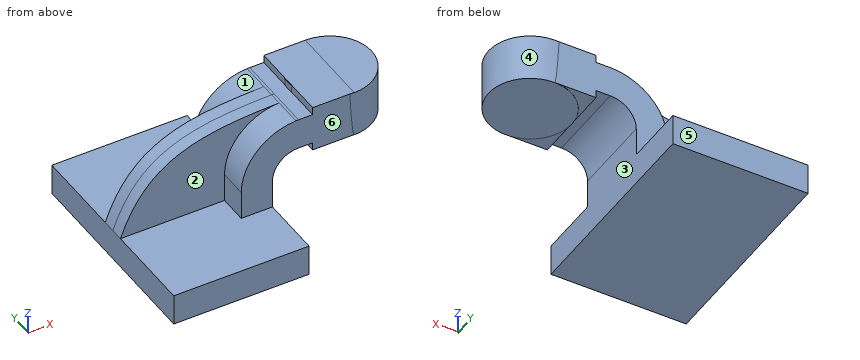
```python
from build123d import *

# Parameters (mm, degrees)
F1_DEPTH = 63.5
F2_DEPTH = 25.4
F3_DEPTH = 7.9375
F4_DEPTH = 25.4


with BuildPart() as f1:
    # F0 (on Front) → F1 (new body, symmetric)
    with BuildSketch(Plane.XZ):
        Polygon((-41.275, -9.525), (41.275, -9.525), (41.275, 9.525), (22.225, 9.525), (-41.275, 9.525), align=None)
    extrude(amount=F1_DEPTH, both=True)

    # F0 (on Front) → F2 (join, symmetric)
    with BuildSketch(Plane.XZ):
        with BuildLine():
            Line((22.225, 9.525), (41.275, 9.525))
            Line((41.275, 9.525), (41.275, 27.0002))
            ThreePointArc((41.275, 27.0002), (45.9246798487, 38.2255201513), (57.15, 42.8752))
            Line((57.15, 42.8752), (65.7820404529, 42.8752))
            Line((65.7820404529, 42.8752), (65.7820404529, 61.9252))
            Line((65.7820404529, 61.9252), (57.15, 61.9252))
            add(Edge.make_bspline(
                [(55.550874855, 61.8885708959), (56.0816141812, 61.9013962884), (56.6146531302, 61.9135944066), (57.15, 61.9252)],
                knots=[110.3600423444, 110.3600423444, 110.3600423444, 110.3600423444, 111.5045361635, 111.5045361635, 111.5045361635, 111.5045361635], degree=3))
            ThreePointArc((55.550874855, 61.8885708959), (31.8952472721, 51.1239038959), (22.225, 27.0002))
            Line((22.225, 27.0002), (22.225, 9.525))
        make_face()
    extrude(amount=F2_DEPTH, both=True)

    # F0 (on Front) → F3 (join, symmetric)
    with BuildSketch(Plane.XZ):
        with BuildLine():
            add(Edge.make_bspline(
                [(-41.275, 9.525), (-25.4220175823, 53.5826509426), (4.3733031342, 60.6518574843), (55.550874855, 61.8885708959)],
                knots=[0, 0, 0, 0, 110.3600423444, 110.3600423444, 110.3600423444, 110.3600423444], degree=3))
            Line((-41.275, 9.525), (22.225, 9.525))
            Line((22.225, 9.525), (22.225, 27.0002))
            ThreePointArc((22.225, 27.0002), (31.8952472721, 51.1239038959), (55.550874855, 61.8885708959))
        make_face()
    extrude(amount=F3_DEPTH, both=True)

    # F0 (on Front) → F4 (join, symmetric)
    with BuildSketch(Plane.XZ):
        Polygon((65.7820404529, 61.9252), (65.7820404529, 42.8752), (65.7820404529, 38.1), (91.1820404529, 38.1), (91.0449102521, 66.675), (65.7820404529, 66.675), align=None)
    extrude(amount=F4_DEPTH, both=True)

    # F0 (on Front) → F5 (revolve)
    with BuildSketch(Plane.XZ):
        Polygon((91.0449102521, 66.675), (91.1820404529, 38.1), (116.5820404529, 38.1), (116.5820404529, 66.675), align=None)
    revolve(axis=Axis((91.1134753525, 0, 52.3875), (-0.0047989019, 0, 0.9999884852)))


solid = f1.part
```
Design review of the part built by this model. Coordinates are the model's own, in mm. Face numbers are marked on the shaded views. A direction names the side the tool comes from. Give positions to 0.01 mm unless a question says otherwise; leave off trailing zeros. Order: outer loops, then holes, each group sorted by start corner. A loop starts at its lowest first (then second) coordinate and runs counter-clockwise, first axis right, second up. Notation, with made-up numbers: (14, 76.25) -> (25, 76.25) arc R5 ccw to (25, 80.25) -> close; hole circle Ø10 at (-32, 21). An arc over 180 degrees is marked (long way). Write item = value, one per line. Start each with the question number.
(1) For the marked faces 1 and 2, list the 3-axis set-ups (+Z, -Z, +X, -X, +Y, -Y) from which the entire face can be reached by the end or side of a thin tool; tool diameter is ignored.
(2) Mouldability with a two-part tool opening along Y and no side actions: class the marked faces 3, 4, 5 and 6 as +Y half, -Y half, draft (parallel to the pull), parting line (faces both ways), or undercut.
(3) We need section A-A on y = 47. Write out the cut boundary in (x, z) (3 decimals), plus the area to 3 significant figures.
(4) To check wall thickness, follow line 1 along Y through (x, z) = (1, 24); line 2 along X through (y, z) = (-8.5, 23) (3 decimals); line 3 along X through (y, z) = (30, 8.5) (3 decimals). State the ranges of each line that lie inside material, in increasing order.
(5) For pin 1 (17 mm diameter, centred on x = 40.5, z = 40, fed in from -Y); pin 2 (5 mm diameter, centred on y = -17, z = 22, fed in from -X) (3 decimals); pin 3 (1.5 mm diameter, centred on x = 20.5, z = 10.5, fed in from +Y), all flat-tipped, find the tip position at first contact; note any pin that passes through.
(6) We need section B-B on z = 1. Write out the cut boundary in (x, y) (3 decimals).
Numbers:
q1.face_1 = +Z, -X, +Y
q1.face_2 = +Z, -X, -Y
q2.face_3 = draft
q2.face_4 = parting line
q2.face_5 = +Y half
q2.face_6 = -Y half
q3.outline = (-41.275, -9.525) -> (41.275, -9.525) -> (41.275, 9.525) -> (-41.275, 9.525) -> close
q3.area = 1,570 mm^2
q4.line_1 = -7.94 to 7.94
q4.line_2 = 22.225 to 41.275
q4.line_3 = -41.275 to 41.275
q5.pin_1 = -25.4
q5.pin_2 = 22.225
q5.pin_3 = 7.94
q6.outline = (-41.275, -63.5) -> (41.275, -63.5) -> (41.275, 63.5) -> (-41.275, 63.5) -> close
